```python
from build123d import *

# Parameters (mm, degrees)
SKETCH_1_W      = 19
SKETCH_1_H      = 19
SKETCH_1_W_2    = 15.88
SKETCH_1_H_2    = 15.88
EXTRUDE_1_DEPTH = 600
FILLET_2_R      = 1


with BuildPart() as part:
    # 스케치1 → 보스-돌출1 (new body)
    with BuildSketch(Plane.XY):
        with Locations((9.5, -9.5)):
            Rectangle(SKETCH_1_W, SKETCH_1_H)
        with Locations((9.5, -9.5)):
            Rectangle(SKETCH_1_W_2, SKETCH_1_H_2, mode=Mode.SUBTRACT)
    extrude(amount=EXTRUDE_1_DEPTH)

    # 필렛2
    fillet_2_edges = [part.edges().sort_by_distance(p)[0] for p in [
        (0, 0, 300),
        (19, 0, 300),
        (19, -19, 300),
        (0, -19, 300),
    ]]
    fillet(fillet_2_edges, radius=FILLET_2_R)


solid = part.part
```
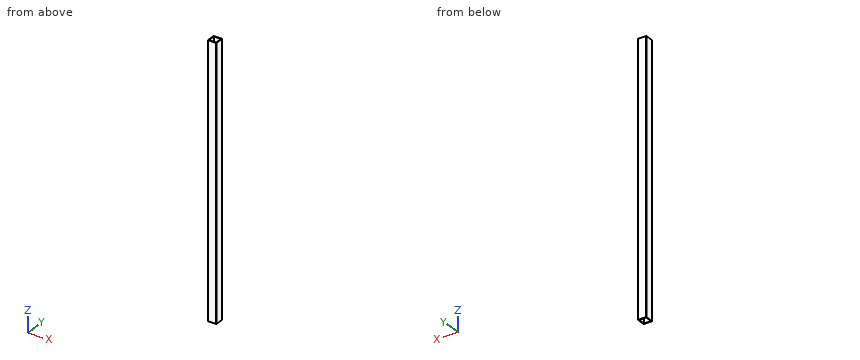
Design review of the part built by this model. Coordinates are the model's own, in mm. Give positions to 0.01 mm unless a question says otherwise; leave off trailing zeros. Write each loop counter-clockwise with the first axis right and the second up, starting at its lowest first coordinate (ties: lowest second). Pieces come first, ordered by that corner, then holes.
(1) Add section A-A (x = 7.25). Give the boundary of the cut face in (y, z).
Checked values:
outline: (-19, 0) - (-17.44, 0) - (-17.44, 600) - (-19, 600) - close; (-1.56, 0) - (0, 0) - (0, 600) - (-1.56, 600) - close
(2) Add section B-B (y = -8). Give the boundary of the cut face in (x, z).
Checked values:
outline: (0, 0) - (1.56, 0) - (1.56, 600) - (0, 600) - close; (17.44, 0) - (19, 0) - (19, 600) - (17.44, 600) - close
(3) Wall thickness on line 1 along Y through (x, z) = (10, 219.5); line 2 along X through (y, z) = (-6.5, 424): over which ranges is each line inside the solid? List them lowest first.
Checked values:
line 1: y = -19 to -17.44, -1.56 to 0
line 2: x = 0 to 1.56, 17.44 to 19
(4) Add section C-C (z = 364). Give the boundary of the cut face in (x, y).
Checked values:
outline: (0, -18) arc R1 ccw to (1, -19) - (18, -19) arc R1 ccw to (19, -18) - (19, -1) arc R1 ccw to (18, 0) - (1, 0) arc R1 ccw to (0, -1) - close; hole (1.56, -17.44) - (17.44, -17.44) - (17.44, -1.56) - (1.56, -1.56) - close
